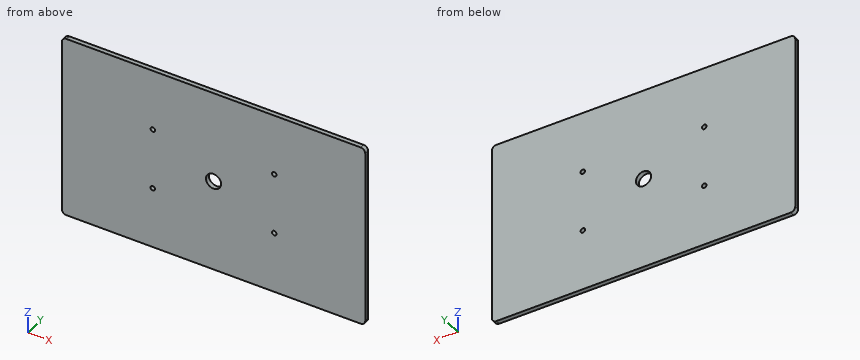
from build123d import *

# Parameters (mm, degrees)
SKETCH1_W               = 200
SKETCH1_H               = 120
BOSS_EXTRUDE1_DEPTH     = 3
FILLET1_R               = 3
SKETCH2_R               = 1.5
CUT_EXTRUDE1_DEPTH      = 3
MIRROR2_COPY_1_SKETCH_R = 1.5
MIRROR2_COPY_1_DEPTH    = 3
SKETCH3_R               = 5
CUT_EXTRUDE2_DEPTH      = 3


with BuildPart() as part:
    # Sketch1 → Boss-Extrude1 (new body)
    with BuildSketch(Plane(origin=(0, 0, 0), x_dir=(1, 0, 0), z_dir=(0, 1, 0))):
        Rectangle(SKETCH1_W, SKETCH1_H)
    extrude(amount=BOSS_EXTRUDE1_DEPTH)

    # Fillet1
    fillet1_edges = [part.edges().sort_by_distance(p)[0] for p in [
        (100, 1.5, 60),
        (-100, 1.5, 60),
        (-100, 1.5, -60),
        (100, 1.5, -60),
    ]]
    fillet(fillet1_edges, radius=FILLET1_R)

    # Sketch2 → Cut-Extrude1 (cut)
    with BuildSketch(Plane(origin=(0, 3, 0), x_dir=(1, 0, 0), z_dir=(0, 1, 0))):
        with Locations((40, 20)):
            Circle(SKETCH2_R)
    cut_extrude1 = extrude(amount=-CUT_EXTRUDE1_DEPTH, mode=Mode.SUBTRACT)

    # Mirror1: Cut-Extrude1 across plane
    add(cut_extrude1.mirror(Plane.XY), mode=Mode.SUBTRACT)

    # Mirror2: Cut-Extrude1 across plane
    add(cut_extrude1.mirror(Plane(origin=(0, 0, 0), x_dir=(0, 0, 1), z_dir=(1, 0, 0))), mode=Mode.SUBTRACT)

    # Mirror2 copy 1 sketch → Mirror2 copy 1 (cut)
    with BuildSketch(Plane(origin=(0, 3, 0), x_dir=(-1, 0, 0), z_dir=(0, 1, 0))):
        with Locations((40, 20)):
            Circle(MIRROR2_COPY_1_SKETCH_R)
    extrude(amount=-MIRROR2_COPY_1_DEPTH, mode=Mode.SUBTRACT)

    # Sketch3 → Cut-Extrude2 (cut)
    with BuildSketch(Plane(origin=(0, 3, 0), x_dir=(1, 0, 0), z_dir=(0, 1, 0))):
        Circle(SKETCH3_R)
    extrude(amount=-CUT_EXTRUDE2_DEPTH, mode=Mode.SUBTRACT)


solid = part.part
Geometry: final body of the model. Coordinates: model frame, mm. Coordinates: 2 decimals unless noted, no trailing zeros. Order: outer loops, then holes, each group sorted by start corner. A loop starts at its lowest first (then second) coordinate and runs counter-clockwise, first axis right, second up. Notation, with made-up numbers: (88, -15) - (147, -15) arc R26 cw to (147, 11) - close; hole circle Ø2 at (-12.5, 88.5). An arc over 180 degrees is marked (long way). Use one line per item in the form item = value.
1) Section A-A (z = 3). Return loops of the section in (x, y), then the cut area to 3 significant figures.
Solutions:
outline = (-100, 0) - (-4, 0) - (-4, 3) - (-100, 3) - close; (4, 0) - (100, 0) - (100, 3) - (4, 3) - close
area = 576 mm^2
2) Ray query, L1, parallel to Z at x = -40, y = 1.85; L2, parallel to X at y = 2.1, z = -20; L3, parallel to X at y = 0.9, z = 0. Return the intervals inside material, ascending.
Solutions:
L1 = -60 to -21.5, -18.5 to 18.5, 21.5 to 60
L2 = -100 to -41.5, -38.5 to 38.5, 41.5 to 100
L3 = -100 to -5, 5 to 100
3) Section B-B (x = 0). Return loops of the section in (y, z).
Solutions:
outline = (0, -60) - (3, -60) - (3, -5) - (0, -5) - close; (0, 5) - (3, 5) - (3, 60) - (0, 60) - close
